Design review of the part shown in the three views and the two pictorial views. Dimensions are in mm from the part's minimum x, y and z. A direction names the side the tool comes from. Give positions to 0.01 mm unless a question says otherwise; leave off trailing zeros. Order: outer loops, then holes, each group sorted by start corner. A loop starts at its lowest first (then second) coordinate and runs counter-clockwise, first axis right, second up. Notation, with made-up numbers: M 17.25,-12 L 45.25,-12 A30 cw 45.25,23 Z; hole C 60.25,22 d1. An arc over 180 degrees is marked long. Answer as a JSON object with one key per item and string values.
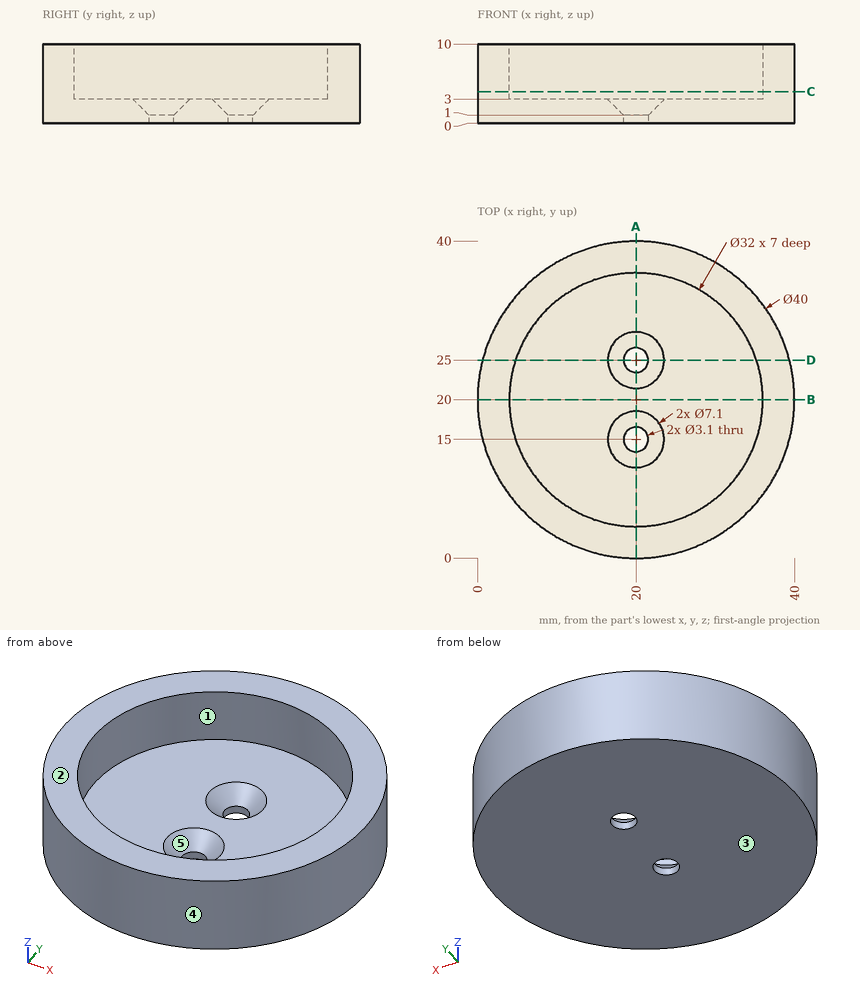
(1) We need section D-D (y = 25). Write out the cut boundary in (x, z).
Checked values:
{"outline": "M 0.64,0 L 18.45,0 L 18.45,1 L 16.45,3 L 4.8,3 L 4.8,10 L 0.64,10 Z; M 21.55,0 L 39.36,0 L 39.36,10 L 35.2,10 L 35.2,3 L 23.55,3 L 21.55,1 Z"}
(2) We need section A-A (x = 20). Write out the cut boundary in (y, z), plus the area to 3 significant figures.
Checked values:
{"outline": "M 0,0 L 13.45,0 L 13.45,1 L 11.45,3 L 4,3 L 4,10 L 0,10 Z; M 16.55,0 L 23.45,0 L 23.45,1 L 21.45,3 L 18.55,3 L 16.55,1 Z; M 26.55,0 L 40,0 L 40,10 L 36,10 L 36,3 L 28.55,3 L 26.55,1 Z", "area": "149 mm^2"}
(3) To check wall thickness, follow L1, parallel to Y at x = 20, z = 0.6; L2, parallel to Z at x = 25.5, y = 17; L3, parallel to Y at x = 20, z = 5.5. State the ranges of each line that lie inside material, in increasing order. Write a range as from..to.
Checked values:
{"L1": "y = 0..13.45, 16.55..23.45, 26.55..40", "L2": "z = 0..3", "L3": "y = 0..4, 36..40"}
(4) Draft analysis for pull direction X (two halves, no side actions). For the marked faces 3, 4 and 5, state which applies: +X half, -X half, draft (parallel to the pull), parting line (faces both ways), or undercut.
Checked values:
{"face 3": "draft", "face 4": "parting line", "face 5": "undercut"}
(5) We need section B-B (y = 20). Write out the cut boundary in (x, z), plus the area to 3 significant figures.
Checked values:
{"outline": "M 0,0 L 40,0 L 40,10 L 36,10 L 36,3 L 4,3 L 4,10 L 0,10 Z", "area": "176 mm^2"}
(6) Insertion check: pin 1 (2 mm diameter, centred on x = 22, z = 3.5, fed in from +Y) (3 decimals); pin 2 (4 mm diameter, centred on x = 16, z = 6, fed in from -Y); pin 3 (1.5 mm diameter, centred on y = 7, z = 4, fed in from +X). Each pin has a flat end and moves straight along its axis. Give the tip position at first contact, or say it passes through.
Checked values:
{"pin 1": "stops at y = 39.975", "pin 2": "stops at y = 0.1", "pin 3": "stops at x = 35.81"}
(7) We need section C-C (z = 4). Write out the cut boundary in (x, y), plus the area to 3 significant figures.
Checked values:
{"outline": "C 20,20 d40; hole C 20,20 d32", "area": "452 mm^2"}
(8) Tool access review of the marked faces 1 and 2: name each direction out of +Z, -Z, +X, -X, +Y, -Y from which nothing blocks a thin tool from reaching the whole face with its end or side.
Checked values:
{"face 1": "+Z", "face 2": "+Z, +X, -X, +Y, -Y"}
